Can you work these out from the model? Positions are in its coordinate system, mm. A direction names the side the tool comes from. Round coordinates to 2 decimals unless told otherwise and drop trailing zeros. Order: outer loops, then holes, each group sorted by start corner. A loop starts at its lowest first (then second) coordinate and runs counter-clockwise, first axis right, second up.
from build123d import *

# Parameters (mm, degrees)
F0_W     = 150.041418
F0_H     = 75.48475
F1_DEPTH = 5
F3_DEPTH = 9.8
F5_DEPTH = 15.9
F6_W     = 48.215222
F6_H     = 44.908039
F7_DEPTH = 12.5
F8_R     = 10
F9_R     = 8


with BuildPart() as f1:
    # F0 (on Top) → F1 (new body)
    with BuildSketch(Plane.XY):
        with Locations((84.918297, -45.505845)):
            Rectangle(F0_W, F0_H)
    extrude(amount=F1_DEPTH)

    # F2 (on face) → F3 (cut)
    with BuildSketch(Plane(origin=(0, 0, 0), x_dir=(1, 0, 0), z_dir=(0, 0, -1))):
        Polygon((144.867465, 78.199215), (144.867465, 83.24822), (134.695292, 83.24822), (134.695292, 43.163463), (144.867465, 43.163463), align=None)
        with BuildLine():
            ThreePointArc((134.695292, 43.163463), (139.781378, 38.077377), (144.867465, 43.163463))
            Line((144.867465, 43.163463), (134.695292, 43.163463))
        make_face()
    extrude(amount=-F3_DEPTH, mode=Mode.SUBTRACT)

    # F4 (on face) → F5 (cut)
    with BuildSketch(Plane.XY.offset(5)):
        Polygon((35.375342, -7.76347), (25.374779, -7.76347), (25.374779, -10.515515), (25.374779, -48.407745), (35.375342, -48.407745), align=None)
        with BuildLine():
            Line((35.375342, -48.407745), (25.374779, -48.407745))
            ThreePointArc((25.374779, -48.407745), (30.375061, -53.408026), (35.375342, -48.407745))
        make_face()
    extrude(amount=-F5_DEPTH, mode=Mode.SUBTRACT)

    # F6 (on face) → F7 (cut)
    with BuildSketch(Plane.XY.offset(5)):
        with Locations((85.245358, -45.718584)):
            Rectangle(F6_W, F6_H)
    extrude(amount=-F7_DEPTH, mode=Mode.SUBTRACT)

    # F8
    f8_edges = [f1.edges().sort_by_distance(p)[0] for p in [
        (109.352969, -23.264565, 2.5),
        (61.137747, -68.172604, 2.5),
        (109.352969, -68.172604, 2.5),
        (61.137747, -23.264565, 2.5),
    ]]
    fillet(f8_edges, radius=F8_R)

    # F9
    f9_edges = [f1.edges().sort_by_distance(p)[0] for p in [
        (9.897588, -7.76347, 2.5),
        (159.939006, -83.24822, 2.5),
    ]]
    fillet(f9_edges, radius=F9_R)


solid = f1.part
(1) Please list where these lines run through material, in increasing order: probe 1 along X at (y, z) = (-36.5, 4); probe 2 along X at (y, z) = (-43.5, 0.5); probe 3 along X at (y, z) = (-71, 1).
(2) I'm going to push a flat-ended pin straight in: pin 1 Ø5 at (x, y) = (138.5, -50.5) entering from +Z. Where does the tip first touch, or does it pass through?
(3) On a 3-axis mill with a long thin cutter (end or side, diameter ignored), from which of +Z, -Z, +X, -X, +Y, -Y can I reach the whole of each face in a straight line? I mean faces 5 (the face through (25.375, -28, 3)), 6 (the face through (22, -7.763, 2)), 7 (the face through (134.695, -63, 2)), 8 (the face through (64.145, -65.321, 2.465)), 9 (the face through (148, -83.248, 2)). Say none if no direction works.
(4) I want a section at C-C, the plane y = -20.5. List the corners of the cut face in (x, z) for me.
(5) I want a section at B-B, the plane z = 3.9. List the corners of the cut face in (x, y) for me.
(6) I want a section at D-D, the plane y = -56.5. List the corners of the cut face in (x, z) for me, plus the area to 3 significant figures.
(7) If we mould it in two halves opening along Y, with no side actions, what happens to faces 1 (the face through (157.5, -81, 2.5)), 2 (the face through (30.265, -53.407, 2.535)), 3 (the face through (144.867, -63, 2)), 4 (the face through (85, -23.265, 3))? For each: pulls with the +Y half, pulls with the -Y half, needs draft (parallel to the pull), parting line crosses it, or undercut.
(8) I want a section at A-A, the plane y = -35. List the corners of the cut face in (x, z) for me, plus the area to 3 significant figures.
Ans:
1. probe 1: x = 9.9 to 25.37, 35.38 to 61.14, 109.35 to 159.94
1. probe 2: x = 9.9 to 25.37, 35.38 to 61.14, 109.35 to 134.7, 144.87 to 159.94
1. probe 3: x = 9.9 to 134.7, 144.87 to 159.94
2. pin 1: passes through
3. face 5: +Z, -Z, +Y
3. face 6: +Z, -Z, +X, -X, +Y
3. face 7: +Z, -Z, -Y
3. face 8: +Z, -Z
3. face 9: +Z, -Z, +X, -X, -Y
4. outline: (9.9, 0) - (25.37, 0) - (25.37, 5) - (9.9, 5) - close; (35.38, 0) - (159.94, 0) - (159.94, 5) - (35.38, 5) - close
5. outline: (9.9, -83.25) - (134.7, -83.25) - (134.7, -43.16) arc R5.09 cw to (144.87, -43.16) - (144.87, -83.25) - (151.94, -83.25) arc R8 ccw to (159.94, -75.25) - (159.94, -7.76) - (35.38, -7.76) - (35.38, -48.41) arc R5 cw to (25.37, -48.41) - (25.37, -7.76) - (17.9, -7.76) arc R8 ccw to (9.9, -15.76) - close; hole (61.14, -58.17) arc R10 ccw to (71.14, -68.17) - (99.35, -68.17) arc R10 ccw to (109.35, -58.17) - (109.35, -33.26) arc R10 ccw to (99.35, -23.26) - (71.14, -23.26) arc R10 ccw to (61.14, -33.26) - close
6. outline: (9.9, 0) - (61.14, 0) - (61.14, 5) - (9.9, 5) - close; (109.35, 0) - (134.7, 0) - (134.7, 5) - (109.35, 5) - close; (144.87, 0) - (159.94, 0) - (159.94, 5) - (144.87, 5) - close
6. area: 458 mm2
7. face 1: pulls with the -Y half
7. face 2: pulls with the +Y half
7. face 3: needs draft
7. face 4: undercut
8. outline: (9.9, 0) - (25.37, 0) - (25.37, 5) - (9.9, 5) - close; (35.38, 0) - (61.14, 0) - (61.14, 5) - (35.38, 5) - close; (109.35, 0) - (159.94, 0) - (159.94, 5) - (109.35, 5) - close
8. area: 459 mm2
